Autodesk Inventor part; units mm, degrees
ref_plane "YZ Plane" through (0, 0, 0) normal (1, 0, 0) x (0, 1, 0)
ref_plane "XZ Plane" through (0, 0, 0) normal (0, 1, 0) x (-1, 0, 0)
ref_plane "XY Plane" through (0, 0, 0) normal (0, 0, 1) x (1, 0, 0)
sketch "Esquisse1" plane through (0, 0, 0) normal (0, 0, 1) x (1, 0, 0)
  circle A0 centre (0, 0) radius 12.5
  dimension "d0" = 25
extrude "Extrusion1" add sketch "Esquisse1" along normal blind 20
shell "Coque1" thickness 1.5 removed faces 1 at (2.488, -2.432, 20)
ref_plane "Plan de construction1" through (0, 0, -20) normal (0, 0, -1) x (-1, 0, 0)
sketch "Esquisse2" plane through (0, 0, -20) normal (0, 0, -1) x (-1, 0, 0)
  circle A0 centre (0, 0) radius 1.5
  dimension "d5" = 3
loft "Lissage1" add profiles "Esquisse2" section 2 edges at (-12.5, 0, 0)
shell "Coque2" thickness 1.5 removed faces 1 at (0.3952, -0.1996, -20)
sketch "Esquisse3" plane through (0, 0, -20) normal (0, 0, -1) x (-1, 0, 0)
  circle A0 centre (0, 0) radius 1.1
  dimension "d11" = 2.2
extrude "Extrusion2" cut sketch "Esquisse3" against normal blind 10
sketch "Esquisse4" plane through (0, 0, 20) normal (0, 0, 1) x (1, 0, 0)
  circle A0 centre (0, 0) radius 12.5
  point P0 (0, -12.5)
ref_plane "Plan de construction2" through (0, -12.5, 20) normal (0, -1, 0) x (1, 0, 0)
sketch "Esquisse5" plane through (0, -12.5, 20) normal (0, -1, 0) x (1, 0, 0)
  circle A0 centre (0, -23.4729) radius 1
  circle A1 centre (0, -23.4729) radius 1.5
  point P0 (0, -20)
  dimension "d14" = 2
  dimension "d15" = 3
extrude "Extrusion3" add sketch "Esquisse5" along normal mid plane 10
sketch "Esquisse6" plane through (0, -17.5, -3.4729) normal (0, -1, 0) x (1, 0, 0)
  circle A0 centre (0, 0) radius 1
  point P0 (0, 3.4729)
extrude "Extrusion4" cut sketch "Esquisse6" against normal blind 15
sketch "Esquisse7" plane through (0, -17.5, -3.4729) normal (0, -1, 0) x (1, 0, 0)
  point P0 (0, 3.4729)
sketch "Esquisse8" plane through (0, -17.5, -3.4729) normal (0, -1, 0) x (1, 0, 0)
  circle A0 centre (0, 0) radius 1
  circle A1 centre (0, 0) radius 2
  point P0 (0, 3.4729)
  dimension "d20" = 4
extrude "Extrusion5" cut sketch "Esquisse8" against normal blind 10
sketch "Esquisse9" plane through (0, 0, 0) normal (0, 0, -1) x (-1, 0, 0)
  circle A0 centre (0, 0) radius 20.0804
extrude "Extrusion6" cut sketch "Esquisse9" against normal blind 20
properties part number "EMBOUT"
Build history of the part. All positions in model axes, mm. Coordinates: 2 decimals unless noted, no trailing zeros. Order: outer loops, then holes, each group sorted by start corner. A loop starts at its lowest first (then second) coordinate and runs counter-clockwise, first axis right, second up. Notation, with made-up numbers: (-34.75, 15) - (1.25, 15) arc R24 ccw to (1.25, 28) - close; hole circle Ø3 at (-15.5, 53.25). An arc over 180 degrees is marked (long way). Write each question's results on one line, items separated by ' | '. Start each with the question number.
Item 1: Mould opens along X. For faces 1 (the face through (-1.05, 0.33, -18.82)), 2 (the face through (1.3, 5.7, -12.1)), 3 (the face through (-2, -9.8, -3.4)), 4 (the face through (11, 0, 0)) say: released by +X, released by -X, zero draft, split by the parting line, or undercut.
Item 2: Band-saw the part on C-C on z = -4. Write the cut outline in (x, y).
Item 3: Band-saw the part on B-B on z = -10. Write the cut outline in (x, y), and give its area (3 significant figures).
Item 4: Flat gauge pins, fed straight in: pin 1 (3 mm diameter, centred on x = 0, z = -3.47, fed in from +Y); pin 2 (6 mm diameter, centred on x = 7, z = -17.5, fed in from +Y); pin 3 (5 mm diameter, centred on x = 0.5, y = 5, fed in from -Z); pin 4 (5 mm diameter, centred on x = -7.5, z = -7.5, fed in from -Y). Where does each tip first touch, or does it go through?
Item 5: Band-saw the part on A-A on x = 0. Write the cut outline in (y, z).
Item 6: Wall check: probe 1 along X at (y, z) = (-6, -7.5); probe 2 along Y at (x, z) = (0, -18.05); probe 3 along Y at (x, z) = (-0.5, -5.5). Give the ranges that are in metal, low to high. Write a range as [from, to].
Numbers:
1) face 1: undercut | face 2: split by the parting line | face 3: undercut | face 4: zero draft
2) outline: (-1.93, -10.12) - (-1.93, -8.37) arc R8.59 cw (long way) to (1.93, -8.37) - (1.93, -10.12) arc R10.3 ccw (long way) to start
3) outline: circle Ø14 at (0, 0); hole circle Ø10.58 at (0, 0) | area: 66.1 mm^2
4) pin 1: y = 11.42 | pin 2: through | pin 3: z = -18.14 | pin 4: y = -7.39
5) outline: (-12.5, 0) - (-11.69, -1.47) - (-9.98, -1.47) - (-10.79, 0) - close; (-9.49, -5.47) - (-1.5, -20) - (-1.1, -20) - (-1.1, -17.61) - (-7.78, -5.47) - close; (1.1, -20) - (1.5, -20) - (12.5, 0) - (10.79, 0) - (1.1, -17.61) - close
6) probe 1: [-5.84, -2.9], [2.9, 5.84] | probe 2: [-2.57, -1.1], [1.1, 2.57] | probe 3: [-9.46, -7.75], [7.75, 9.46]
